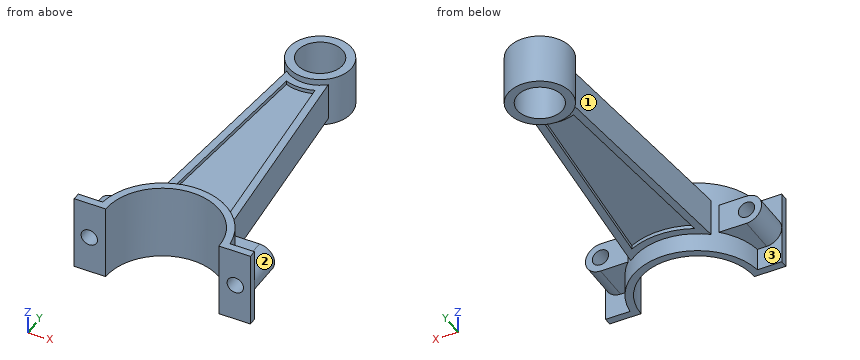
from build123d import *

# Parameters (mm, degrees)
BOSS_EXTRUDE3_DEPTH = 15
BOSS_EXTRUDE4_DEPTH = 6
BOSS_EXTRUDE5_DEPTH = 7.5
BOSS_EXTRUDE6_DEPTH = 10
CUT_EXTRUDE2_DEPTH  = 15
SKETCH3_7_R         = 3.2500000000000004
SKETCH3_7_R_2       = 3.2499999999999973
CUT_EXTRUDE3_DEPTH  = 119.20156513346176
CUT_EXTRUDE5_DEPTH  = 1.5
CUT_EXTRUDE6_START  = -1.5
CUT_EXTRUDE6_DEPTH  = 1.5


with BuildPart() as part:
    # Sketch1 → Boss-Extrude3 (new, symmetric)
    with BuildSketch(Plane.XY):
        with BuildLine():
            ThreePointArc((-3.384e-13, -91.9), (-8.457393215406437, -93.34334811325573), (-15.957377604105265, -97.51000000000002))
            ThreePointArc((-15.957377604105265, -97.51000000000002), (-17.03611469018102, -98.42578601725495), (-18.06239186818843, -99.4))
            ThreePointArc((-18.06239186818843, -99.4), (-22.95258596956737, -106.29014863692505), (-25.32291452420118, -114.40000000000002))
            Line((-25.322914524201185, -114.40000000000002), (-28.999999999999986, -114.40000000000002))
            Line((-28.999999999999986, -114.40000000000002), (-28.999999999999986, -117.40000000000002))
            Line((-28.999999999999986, -117.4), (-22.499999999999982, -117.4))
            ThreePointArc((-22.499999999999982, -117.4), (-15.909902576697428, -101.49009742330281), (-3.4057e-13, -94.9))
            Line((1.352e-14, -94.9), (1.315e-14, -91.9))
        make_face()
        with BuildLine():
            ThreePointArc((18.062391868188463, -99.4), (17.036114690181044, -98.42578601725495), (15.957377604105286, -97.51000000000002))
            ThreePointArc((15.957377604105286, -97.51000000000002), (8.457393215406128, -93.34334811325562), (-3.384e-13, -91.9))
            Line((1.315e-14, -91.9), (1.352e-14, -94.9))
            ThreePointArc((-3.4557e-13, -94.9), (15.909902576697208, -101.49009742330256), (22.500000000000018, -117.4))
            Line((22.500000000000018, -117.4), (29.000000000000018, -117.4))
            Line((29.000000000000018, -117.40000000000002), (29.000000000000018, -114.40000000000002))
            Line((29.000000000000018, -114.40000000000002), (25.32291452420122, -114.40000000000002))
            ThreePointArc((25.32291452420122, -114.40000000000002), (22.9525859695674, -106.29014863692505), (18.062391868188463, -99.4))
        make_face()
        Polygon((35.000000000000014, -114.40000000000002), (29.000000000000018, -114.40000000000002), (29.000000000000018, -117.40000000000002), (35.000000000000014, -117.4), align=None)
        Polygon((-28.999999999999986, -117.40000000000002), (-28.999999999999986, -114.40000000000002), (-34.99999999999999, -114.40000000000002), (-34.99999999999999, -117.4), align=None)
    extrude(amount=BOSS_EXTRUDE3_DEPTH, both=True)

    # Sketch1_6 → Boss-Extrude4 (add, symmetric)
    with BuildSketch(Plane.XY):
        with BuildLine():
            ThreePointArc((-25.32291452420118, -114.40000000000002), (-22.95258596956737, -106.29014863692505), (-18.06239186818843, -99.4))
            Line((-18.062391868188435, -99.4), (-28.99999999999999, -99.4))
            Line((-28.99999999999999, -99.4), (-28.999999999999986, -114.40000000000002))
            Line((-28.999999999999986, -114.40000000000002), (-25.322914524201185, -114.40000000000002))
        make_face()
        Polygon((-28.999999999999986, -114.40000000000002), (-28.99999999999999, -99.4), (-34.99999999999999, -99.4), (-34.99999999999999, -114.40000000000002), align=None)
        with BuildLine():
            Line((29.000000000000014, -99.4), (18.062391868188463, -99.4))
            ThreePointArc((18.062391868188463, -99.4), (22.9525859695674, -106.29014863692505), (25.32291452420122, -114.40000000000002))
            Line((25.32291452420122, -114.40000000000002), (29.000000000000018, -114.40000000000002))
            Line((29.000000000000018, -114.40000000000002), (29.000000000000014, -99.4))
        make_face()
        Polygon((35.000000000000014, -99.4), (29.000000000000014, -99.4), (29.000000000000018, -114.40000000000002), (35.000000000000014, -114.40000000000002), align=None)
    extrude(amount=BOSS_EXTRUDE4_DEPTH, both=True)

    # Sketch1_7 → Boss-Extrude5 (add, symmetric)
    with BuildSketch(Plane.XY):
        with BuildLine():
            ThreePointArc((-3.4647e-13, -12.5), (-4.407030277273776, -11.697353723607414), (-8.248094723826778, -9.392493461630988))
            Line((-8.248094723826776, -9.392493461630991), (-15.957377604105261, -97.51000000000002))
            ThreePointArc((-15.957377604105265, -97.51000000000002), (-8.457393215406437, -93.34334811325573), (-3.384e-13, -91.9))
            Line((1.315e-14, -91.9), (3.43e-15, -12.5))
        make_face()
        with BuildLine():
            Line((15.957377604105288, -97.51000000000002), (8.248094723826782, -9.392493461630991))
            ThreePointArc((8.248094723826778, -9.392493461630988), (4.407030277273449, -11.697353723607536), (-3.4647e-13, -12.5))
            Line((3.43e-15, -12.5), (1.315e-14, -91.9))
            ThreePointArc((-3.384e-13, -91.9), (8.457393215406128, -93.34334811325562), (15.957377604105286, -97.51000000000002))
        make_face()
    extrude(amount=BOSS_EXTRUDE5_DEPTH, both=True)

    # Sketch1_8 → Boss-Extrude6 (add, symmetric)
    with BuildSketch(Plane.XY):
        with BuildLine():
            ThreePointArc((12.5, 0), (8.838834764831827, 8.838834764831862), (-4.919e-14, 12.5))
            Line((3.7e-16, 12.5), (8e-16, 9.000000000000002))
            ThreePointArc((1.3644e-13, 9.000000000000002), (6.363961030678977, 6.3639610306788805), (9.000000000000002, 0))
            ThreePointArc((9.000000000000002, -2.2e-15), (6.363961030678978, -6.36396103067888), (1.4223e-13, -9.000000000000002))
            Line((3e-15, -9), (3.43e-15, -12.5))
            ThreePointArc((-3.4647e-13, -12.5), (4.407030277273449, -11.697353723607536), (8.248094723826778, -9.392493461630988))
            ThreePointArc((8.248094723826778, -9.392493461630988), (11.387519133855156, -5.155037145945963), (12.5, -3.06e-15))
        make_face()
        with BuildLine():
            Line((8e-16, 9.000000000000002), (3.7e-16, 12.5))
            ThreePointArc((-4.919e-14, 12.5), (-11.697353723607485, 4.407030277273588), (-8.248094723826778, -9.392493461630988))
            ThreePointArc((-8.248094723826778, -9.392493461630988), (-4.407030277273776, -11.697353723607414), (-3.4647e-13, -12.5))
            Line((3.43e-15, -12.5), (3e-15, -9))
            ThreePointArc((1.4223e-13, -9.000000000000002), (-9.000000000000002, -2.89e-15), (1.3644e-13, 9.000000000000002))
        make_face()
    extrude(amount=BOSS_EXTRUDE6_DEPTH, both=True)

    # Sketch3 → Cut-Extrude2 (cut)
    with BuildSketch(Plane(origin=(0, -99.4, 0), x_dir=(1, 0, 0), z_dir=(0, 1, 0))):
        with BuildLine():
            Line((-35.000000000000014, 6.22e-15), (-35.000000000000014, -6))
            Line((-35.000000000000014, -6), (-29, -6.000000000000013))
            ThreePointArc((-29, -6.000000000000013), (-33.2426406871193, -4.2426406871192945), (-35.000000000000014, 7.3e-16))
        make_face()
        with BuildLine():
            Line((-35.000000000000014, 6), (-35.000000000000014, 6.22e-15))
            ThreePointArc((-35.000000000000014, 7.3e-16), (-33.24264068711929, 4.2426406871192945), (-29, 6.000000000000013))
            Line((-29, 6.000000000000013), (-35.000000000000014, 6))
        make_face()
        with BuildLine():
            Line((35.000000000000014, 6), (29, 6.000000000000013))
            ThreePointArc((29, 6.000000000000013), (33.24264068711929, 4.2426406871192945), (35.000000000000014, 0))
            Line((35.000000000000014, 0), (35.000000000000014, 6))
        make_face()
        with BuildLine():
            ThreePointArc((35.000000000000014, -1.47e-15), (33.24264068711929, -4.242640687119295), (29, -6.000000000000013))
            Line((29, -6.000000000000013), (35.000000000000014, -6))
            Line((35.000000000000014, -6), (35.000000000000014, 0))
        make_face()
    extrude(amount=-CUT_EXTRUDE2_DEPTH, mode=Mode.SUBTRACT)

    # Sketch3_7 → Cut-Extrude3 (cut, through all)
    with BuildSketch(Plane(origin=(0, -99.4, 0), x_dir=(1, 0, 0), z_dir=(0, 1, 0))):
        with Locations(Location((-29, 0, 0), (0, 0, 270))):
            Circle(SKETCH3_7_R)
        with Locations(Location((29, 0, 0), (0, 0, 270))):
            Circle(SKETCH3_7_R_2)
    extrude(amount=-CUT_EXTRUDE3_DEPTH, mode=Mode.SUBTRACT)

    # Sketch4 → Cut-Extrude5 (cut)
    with BuildSketch(Plane.XY.offset(7.5)):
        with BuildLine():
            Line((5.6767522219735, -14.423053914144496), (12.442830342322818, -91.75968071430914))
            ThreePointArc((12.442830342322818, -91.75968071430914), (1.802e-14, -88.9), (-12.44283034232279, -91.75968071430914))
            Line((-12.44283034232279, -91.75968071430914), (-5.676752221973489, -14.4230539141445))
            ThreePointArc((-5.676752221973489, -14.4230539141445), (7.83e-15, -15.499999999999998), (5.6767522219735, -14.423053914144496))
        make_face()
    extrude(amount=-CUT_EXTRUDE5_DEPTH, mode=Mode.SUBTRACT)

    # Sketch6 → Cut-Extrude6 (cut)
    with BuildSketch(Plane(origin=(0, 0, -7.5), x_dir=(-1, 0, 0), z_dir=(0, 0, -1)).offset(CUT_EXTRUDE6_START)):
        with BuildLine():
            Line((5.67675222197347, -14.423053914144495), (12.442830342322795, -91.75968071430914))
            ThreePointArc((12.442830342322795, -91.75968071430914), (-7.36e-15, -88.9), (-12.442830342322805, -91.75968071430914))
            Line((-12.442830342322805, -91.75968071430914), (-5.676752221973512, -14.423053914144502))
            ThreePointArc((-5.676752221973512, -14.423053914144502), (-1.862e-14, -15.499999999999998), (5.67675222197347, -14.423053914144495))
        make_face()
    extrude(amount=CUT_EXTRUDE6_DEPTH, mode=Mode.SUBTRACT)


solid = part.part
Read the model definition and answer for the solid it produces. Units are mm, in the model's axes. Face numbers are marked on the shaded views. A direction names the side the tool comes from. Coordinates: 2 decimals unless noted, no trailing zeros. Write each loop counter-clockwise with the first axis right and the second up, starting at its lowest first coordinate (ties: lowest second). Pieces come first, ordered by that corner, then holes. Notation, with made-up numbers: (-34, -2.5) -> (-10, -2.5) arc R15 ccw to (-10, 15.5) -> close; hole circle Ø7 at (-37, -15.75). An arc over 180 degrees is marked (long way). Return JSON: item names as keys, results as strings.
(1) The part is cut by section B-B on x = 0. Give the vertices of the cut face in (y, z).
Answers below:
{"outline": "(-94.9, -15) -> (-91.9, -15) -> (-91.9, -7.5) -> (-88.9, -7.5) -> (-88.9, -6) -> (-15.5, -6) -> (-15.5, -7.5) -> (-12.5, -7.5) -> (-12.5, -10) -> (-9, -10) -> (-9, 10) -> (-12.5, 10) -> (-12.5, 7.5) -> (-15.5, 7.5) -> (-15.5, 6) -> (-88.9, 6) -> (-88.9, 7.5) -> (-91.9, 7.5) -> (-91.9, 15) -> (-94.9, 15) -> close; (9, -10) -> (12.5, -10) -> (12.5, 10) -> (9, 10) -> close"}
(2) The part is cut by section A-A on y = 0. Give the vertices of the cut face in (x, z), then the cut area to 3 significant figures.
Answers below:
{"outline": "(-12.5, -10) -> (-9, -10) -> (-9, 10) -> (-12.5, 10) -> close; (9, -10) -> (12.5, -10) -> (12.5, 10) -> (9, 10) -> close", "area": "140 mm^2"}
(3) Consider line 1 along X through (y, z) = (0, 3); line 2 along X through (y, z) = (-105, 0); line 3 along X through (y, z) = (-111.5, 0). Determine where each line is inside the solid, lowest interval first. Write a range as from..to.
Answers below:
{"line 1": "-12.5..-9, 9..12.5", "line 2": "-35..-32.25, -25.75..-18.77, 18.77..25.75, 32.25..35", "line 3": "-35..-32.25, -25.75..-21.71, 21.71..25.75, 32.25..35"}
(4) The part is cut by section D-D on x = 14. Give the vertices of the cut face in (y, z), then the cut area to 3 significant figures.
Answers below:
{"outline": "(-99.79, -15) -> (-96.09, -15) -> (-96.09, -7.5) -> (-75.14, -7.5) -> (-75.14, 7.5) -> (-96.09, 7.5) -> (-96.09, 15) -> (-99.79, 15) -> close", "area": "425 mm^2"}
(5) The part is cut by section C-C on y = -61.5. Give the vertices of the cut face in (x, z), then the cut area to 3 significant figures.
Answers below:
{"outline": "(-12.81, -7.5) -> (-9.8, -7.5) -> (-9.8, -6) -> (9.8, -6) -> (9.8, -7.5) -> (12.81, -7.5) -> (12.81, 7.5) -> (9.8, 7.5) -> (9.8, 6) -> (-9.8, 6) -> (-9.8, 7.5) -> (-12.81, 7.5) -> close", "area": "325 mm^2"}
(6) Which of the six approach directions +Z, -Z, +X, -X, +Y, -Y give full straight-line access (tool end or side, diameter ignored) to the marked faces 1, 2 and 3?
Answers below:
{"face 1": "+Z, -Z, -X", "face 2": "+X, +Y", "face 3": "-Z, -X, +Y"}
(7) Each of these flat-tipped pins is pushed along its axis until it touches: P1, Ø6, axis at x = 14, y = -74.5, coming from the -Z side; P2, Ø12, axis at x = -28, z = 3.5, coming from the +Y side; P3, Ø6, axis at y = -58, z = 2, coming from the -X side. Where does it stop, or does it pass through?
Answers below:
{"P1": "z = -7.5", "P2": "y = -99.4", "P3": "x = -12.76"}
